```python
from build123d import *

# Parameters (mm, degrees)
CYLINDER003_R           = 10.2
CYLINDER003_DEPTH       = 20
CYLINDER003_PITCH_ANGLE = 90
CYLINDER_R              = 11.2
CYLINDER_DEPTH          = 7.2
CYLINDER_ROLL_ANGLE     = -90
CYLINDER005_R           = 2
CYLINDER005_DEPTH       = 30
BOX_W                   = 30.2
BOX_H                   = 7.2
BOX_DEPTH               = 24
CYLINDER004_R           = 8
CYLINDER004_DEPTH       = 30
CYLINDER004_ROLL_ANGLE  = -90
CYLINDER002_R           = 14
CYLINDER002_DEPTH       = 24
CYLINDER002_PITCH_ANGLE = 90
BOX001_W                = 30
BOX001_H                = 11
BOX001_DEPTH            = 30
CYLINDER001_R           = 15
CYLINDER001_DEPTH       = 15
CYLINDER001_ROLL_ANGLE  = -90


with BuildPart() as pipe:
    # Cylinder003 → Cylinder003 (new body)
    with BuildSketch(Plane.XY):
        Circle(CYLINDER003_R)
    extrude(amount=CYLINDER003_DEPTH)


with BuildPart() as pipe_1:
    # Cylinder003 pitch: moved
    add(pipe.part.rotate(Axis((0, 0, 0), (0, 1, 0)), CYLINDER003_PITCH_ANGLE))


with BuildPart() as pipe_2:
    # Cylinder003 placement: moved
    add(pipe_1.part.moved(Location((-30, 0, 0))))


with BuildPart() as bearing:
    # Cylinder → Cylinder (new body)
    with BuildSketch(Plane.XY):
        Circle(CYLINDER_R)
    extrude(amount=CYLINDER_DEPTH)


with BuildPart() as bearing_1:
    # Cylinder roll: moved
    add(bearing.part.rotate(Axis((0, 0, 0), (1, 0, 0)), CYLINDER_ROLL_ANGLE))


with BuildPart() as bearing_2:
    # Cylinder placement: moved
    add(bearing_1.part.moved(Location((0, -3.6, 0))))


with BuildPart() as cylinder003:
    # Cylinder005 → Cylinder005 (new body)
    with BuildSketch(Plane(origin=(-20, 0, -15), x_dir=(1, 0, 0), z_dir=(0, 0, 1))):
        Circle(CYLINDER005_R)
    extrude(amount=CYLINDER005_DEPTH)


with BuildPart() as cube:
    # Box → Box (new body)
    with BuildSketch(Plane(origin=(-30, -3.6, -12), x_dir=(1, 0, 0), z_dir=(0, 0, 1))):
        with Locations((15.1, 3.6)):
            Rectangle(BOX_W, BOX_H)
    extrude(amount=BOX_DEPTH)


with BuildPart() as negative_fusion:
    # Cylinder004 → Cylinder004 (new body)
    with BuildSketch(Plane.XY):
        Circle(CYLINDER004_R)
    extrude(amount=CYLINDER004_DEPTH)


with BuildPart() as negative_fusion_1:
    # Cylinder004 roll: moved
    add(negative_fusion.part.rotate(Axis((0, 0, 0), (1, 0, 0)), CYLINDER004_ROLL_ANGLE))


with BuildPart() as negative_fusion_2:
    # Cylinder004 placement: moved
    add(negative_fusion_1.part.moved(Location((0, -15, 0))))

    # Fusion001: union Pipe, Bearing, Cylinder003, Cube
    add(pipe_2.part)
    add(bearing_2.part)
    add(cylinder003.part)
    add(cube.part)


with BuildPart() as cylinder002:
    # Cylinder002 → Cylinder002 (new body)
    with BuildSketch(Plane.XY):
        Circle(CYLINDER002_R)
    extrude(amount=CYLINDER002_DEPTH)


with BuildPart() as cylinder002_1:
    # Cylinder002 pitch: moved
    add(cylinder002.part.rotate(Axis((0, 0, 0), (0, 1, 0)), CYLINDER002_PITCH_ANGLE))


with BuildPart() as cylinder002_2:
    # Cylinder002 placement: moved
    add(cylinder002_1.part.moved(Location((-30, 0, 0))))


with BuildPart() as cube001:
    # Box001 → Box001 (new body)
    with BuildSketch(Plane(origin=(-30, -5.5, -15), x_dir=(1, 0, 0), z_dir=(0, 0, 1))):
        with Locations((15, 5.5)):
            Rectangle(BOX001_W, BOX001_H)
    extrude(amount=BOX001_DEPTH)


with BuildPart() as cut:
    # Cylinder001 → Cylinder001 (new body)
    with BuildSketch(Plane.XY):
        Circle(CYLINDER001_R)
    extrude(amount=CYLINDER001_DEPTH)


with BuildPart() as cut_1:
    # Cylinder001 roll: moved
    add(cut.part.rotate(Axis((0, 0, 0), (1, 0, 0)), CYLINDER001_ROLL_ANGLE))


with BuildPart() as cut_2:
    # Cylinder001 placement: moved
    add(cut_1.part.moved(Location((0, -7.5, 0))))

    # Fusion: union Cylinder002, Cube001
    add(cylinder002_2.part)
    add(cube001.part)

    # Cut: cut Negative Fusion
    add(negative_fusion_2.part, mode=Mode.SUBTRACT)


solid = cut_2.part
```
Could you check a few things on this model? Use its own coordinates, in mm. A direction names the side the tool comes from. Give positions to 0.01 mm unless a question says otherwise; leave off trailing zeros. Loops run counter-clockwise (first coordinate to the right, second up) from the corner with the lowest first, then second, coordinate; pieces in that order, holes last. Notation, with made-up numbers: (-30, 31) - (7, 31) arc R7 cw to (7, 36) - close; hole circle Ø7 at (84, -16.5). An arc over 180 degrees is marked (long way). Answer in a Markdown table with one row per item. Add a question column.
Q1. If we section it at B-B (x = -10.5): List the corners of the cut face in (y, z) for me, plus the area to 3 significant figures.
Q2. If we section it at A-A (z = 0): List the corners of the cut face in (x, y) for me.
Q3. Which directions (+Z, -Z, +X, -X, +Y, -Y) give clear straight access to the entire face, cutting with the end or side of a thin tool? Please do faces 5 (the face through (-18, 14, 0)), 6 (the face through (-6, 10, 8)), 7 (the face through (11.2, -0.1, 0.2)), 8 (the face through (-19, 5.5, -14)).
Q4. For pin 1 (2.5 mm diameter, centred on y = 11.5, z = -7.5, fed in from +X); pin 2 (1.7 mm diameter, centred on x = -18, z = 14.5, fed in from -Y); pin 3 (12 mm diameter, centred on x = 5.5, z = -6, fed in from -Y), each with a flat end and sliding along its axis, tell me the tip position at first contact or that it passes through.
Q5. We'd pull the mould along Y, two halves only. Please class faces 1 (the face through (-6, -10, 8)), 2 (the face through (-18, -14, 0)), 3 (the face through (-20.1, 10.2, -0.2)), 4 (the face through (8, 7.5, 3)): +Y half, -Y half, draft (parallel to the pull), parting line (faces both ways), or undercut.
Q6. If we section it at D-D (x = -20): List the corners of the cut face in (y, z) for me.
Q7. Please list where these lines run through material, in increasing order: L1, parallel to Z at x = -26, y = 2; L2, parallel to Z at x = 0, y = 7; L3, parallel to Y at x = 5.5, z = 7. Write a range as from..to.
The answers:
| question | item | result |
|---|---|---|
| 1 | outline | (-5.5, -15) - (5.5, -15) - (5.5, -12.87) arc R14 ccw to (5.5, 12.87) - (5.5, 15) - (-5.5, 15) - (-5.5, 12.87) arc R14 ccw to (-5.5, -12.87) - close; hole (-3.6, -12) - (3.6, -12) - (3.6, -9.54) arc R10.2 ccw to (3.6, 9.54) - (3.6, 12) - (-3.6, 12) - (-3.6, 9.54) arc R10.2 ccw to (-3.6, -9.54) - close |
| 1 | area | 290 mm^2 |
| 2 | outline | (-30, -14) - (-8, -14) - (-8, -3.6) - (-10, -3.6) - (-10, -10.2) - (-30, -10.2) - close; (-30, 10.2) - (-10, 10.2) - (-10, 3.6) - (-8, 3.6) - (-8, 14) - (-30, 14) - close; (8, -7.5) - (15, -7.5) - (15, 7.5) - (8, 7.5) - (8, 3.6) - (11.2, 3.6) - (11.2, -3.6) - (8, -3.6) - close |
| 3 | face 5 | -X, +Y |
| 3 | face 6 | +Z, -Z, +X, +Y |
| 3 | face 7 | -X |
| 3 | face 8 | -Z, -X, +Y |
| 4 | pin 1 | stops at x = -6 |
| 4 | pin 2 | stops at y = -5.5 |
| 4 | pin 3 | stops at y = -7.5 |
| 5 | face 1 | draft |
| 5 | face 2 | -Y half |
| 5 | face 3 | undercut |
| 5 | face 4 | +Y half |
| 6 | outline | (-5.5, -15) - (-2, -15) - (-2, -12) - (-3.6, -12) - (-3.6, -9.54) arc R10.2 cw to (-3.6, 9.54) - (-3.6, 12) - (-2, 12) - (-2, 15) - (-5.5, 15) - (-5.5, 12.87) arc R14 ccw to (-5.5, -12.87) - close; (2, -15) - (5.5, -15) - (5.5, -12.87) arc R14 ccw to (5.5, 12.87) - (5.5, 15) - (2, 15) - (2, 12) - (3.6, 12) - (3.6, 9.54) arc R10.2 cw to (3.6, -9.54) - (3.6, -12) - (2, -12) - close |
| 7 | L1 | z = -15..-12, 12..15 |
| 7 | L2 | z = -15..-8, 8..15 |
| 7 | L3 | y = -7.5..-3.6, 3.6..7.5 |
